Source: CAD feature listing. Evaluate the final solid. Frame: model axes, mm. A direction names the side the tool comes from. Give positions to 0.01 mm unless a question says otherwise; leave off trailing zeros. Return JSON: item names as keys, results as strings. Group by question number.
(1) Access query for faces 1 (the face through (21.5, 2, 22)), 2 (the face through (60, 2, -31)), 3 (the face through (-8, 2, -27.5)), 4 (the face through (-105, 2, -27.5)). Directions: +Z, -Z, +X, -X, +Y, -Y. A direction counts if a zero-diameter tool reaches every point of the face in a straight line with its end or side. Return the directions, or none.
(2) Draft query along Z for faces 5 (the face through (105, 2, 27.5)), 6 (the face through (60, 2, 32)), 7 (the face through (3.859, 2.348, 26.297)). Return one class per face: released by +Z, released by -Z, zero draft, split by the parting line, or undercut.
(3) Cut plane A-A on y = 1.25. Give the number of separate pieces and of enclosed holes in the cut face, then the cut area to 3 significant figures.
(4) Ray query, line 1 (Z direction, x = 56, y = 1.6); line 2 (Z direction, x = -16, y = 4.1); line 3 (X direction, y = 1.85, z = 32.5). Return the intervals inside material, ascending. Write a range as from..to.
(5) Pin query (flat end, axial travel): pin 1 (5 mm diameter, centred on x = 85, z = -5.5, fed in from -Y); pin 2 (1.4 mm diameter, centred on y = 3, z = 35, fed in from -X); pin 3 (2.5 mm diameter, centred on x = -104, y = 3.5, fed in from +Z). Return the tip coordinate at first contact, or that it passes through.
```python
from build123d import *

# Parameters (mm, degrees)
SKETCH1_R           = 1.45
BOSS_EXTRUDE1_DEPTH = 4.7625
SKETCH2_R           = 1.45
SKETCH2_R_2         = 1.6
SKETCH2_R_3         = 2.25
SKETCH2_R_4         = 1.5625
SKETCH2_W           = 25
SKETCH2_H           = 22.5
CUT_EXTRUDE1_DEPTH  = 5.7625
SKETCH3_R           = 0.5
CUT_EXTRUDE2_DEPTH  = 5.7625
FILLET1_R           = 4


with BuildPart() as part:
    # Sketch1 → Boss-Extrude1 (new body)
    with BuildSketch(Plane(origin=(0, 0, 0), x_dir=(1, 0, 0), z_dir=(0, 1, 0))):
        Polygon((100, 37.5), (100, 27.5), (110, 27.5), (110, -27.5), (100, -27.5), (100, -37.5), (-100, -37.5), (-100, -27.5), (-110, -27.5), (-110, 27.5), (-100, 27.5), (-100, 37.5), align=None)
        with Locations((-95, 32.5)):
            Circle(SKETCH1_R, mode=Mode.SUBTRACT)
        with Locations((-105, 22.5)):
            Circle(SKETCH1_R, mode=Mode.SUBTRACT)
        with Locations((105, 22.5)):
            Circle(SKETCH1_R, mode=Mode.SUBTRACT)
        with Locations((95, 32.5)):
            Circle(SKETCH1_R, mode=Mode.SUBTRACT)
        with Locations((-105, -22.5)):
            Circle(SKETCH1_R, mode=Mode.SUBTRACT)
        with Locations((-95, -32.5)):
            Circle(SKETCH1_R, mode=Mode.SUBTRACT)
        with Locations((95, -32.5)):
            Circle(SKETCH1_R, mode=Mode.SUBTRACT)
        with Locations((105, -22.5)):
            Circle(SKETCH1_R, mode=Mode.SUBTRACT)
    extrude(amount=BOSS_EXTRUDE1_DEPTH)

    # Sketch2 → Cut-Extrude1 (cut, through all)
    with BuildSketch(Plane(origin=(0, 4.7625, 0), x_dir=(1, 0, 0), z_dir=(0, 1, 0))):
        with Locations((-25, -22.5)):
            Circle(SKETCH2_R)
        with Locations((-25, 22.5)):
            Circle(SKETCH2_R)
        with Locations((-91.76, -24.96)):
            Circle(SKETCH2_R_2)
        with Locations((-93.03, 23.3)):
            Circle(SKETCH2_R_2)
        with Locations((-40.96, -9.72)):
            Circle(SKETCH2_R_2)
        with Locations((-40.96, 18.22)):
            Circle(SKETCH2_R_2)
        with Locations((45, 5.5)):
            Circle(SKETCH2_R_3)
        with Locations((65, 5.5)):
            Circle(SKETCH2_R_3)
        with Locations((85, 5.5)):
            Circle(SKETCH2_R_3)
        with Locations((56, -21.5)):
            Circle(SKETCH2_R_4)
        with Locations((94, -21.5)):
            Circle(SKETCH2_R_4)
        with Locations((94, 21.5)):
            Circle(SKETCH2_R_4)
        with Locations((56, 21.5)):
            Circle(SKETCH2_R_4)
        Polygon((16.075, 3.65), (23.925, 3.65), (23.925, -7.65), (21.5, -7.65), (21.5, -37.5), (18.5, -37.5), (18.5, -7.65), (16.075, -7.65), align=None)
        with BuildLine():
            Line((70, 37.5), (70, 25.5))
            ThreePointArc((70, 25.5), (65, 20.5), (60, 25.5))
            Line((60, 25.5), (60, 37.5))
            ThreePointArc((60, 37.5), (65, 42.5), (70, 37.5))
        make_face()
        with BuildLine():
            Line((60, -37.5), (60, -25.5))
            ThreePointArc((60, -25.5), (65, -20.5), (70, -25.5))
            Line((70, -25.5), (70, -37.5))
            ThreePointArc((70, -37.5), (65, -42.5), (60, -37.5))
        make_face()
        with Locations((-7.5, -16.25)):
            Rectangle(SKETCH2_W, SKETCH2_H)
        with Locations((-7.5, 16.25)):
            Rectangle(SKETCH2_W, SKETCH2_H)
        with BuildLine():
            Line((-70, -37.5), (-70, -17.5))
            ThreePointArc((-70, -17.5), (-60, -7.5), (-50, -17.5))
            Line((-50, -17.5), (-50, -37.5))
            ThreePointArc((-50, -37.5), (-60, -47.5), (-70, -37.5))
        make_face()
    extrude(amount=-CUT_EXTRUDE1_DEPTH, mode=Mode.SUBTRACT)

    # Sketch3 → Cut-Extrude2 (cut, through all)
    with BuildSketch(Plane(origin=(0, 4.7625, 0), x_dir=(1, 0, 0), z_dir=(0, 1, 0))):
        with Locations((-100.25, 27.75)):
            Circle(SKETCH3_R)
        with Locations((-100.25, -27.75)):
            Circle(SKETCH3_R)
        with Locations((100.25, -27.75)):
            Circle(SKETCH3_R)
        with Locations((100.25, 27.75)):
            Circle(SKETCH3_R)
    extrude(amount=-CUT_EXTRUDE2_DEPTH, mode=Mode.SUBTRACT)

    # Fillet1
    fillet1_edges = [part.edges().sort_by_distance(p)[0] for p in [
        (-20, 2.38125, 27.5),
        (-20, 2.38125, 5),
        (5, 2.38125, 5),
        (5, 2.38125, 27.5),
        (-20, 2.38125, -5),
        (-20, 2.38125, -27.5),
        (5, 2.38125, -27.5),
        (5, 2.38125, -5),
    ]]
    fillet(fillet1_edges, radius=FILLET1_R)


solid = part.part
```
Answers:
{
 "1": {"face 1": "+Z, +Y, -Y", "face 2": "-Z, +Y, -Y", "face 3": "+Y, -Y", "face 4": "-Z, -X, +Y, -Y"},
 "2": {"face 5": "released by +Z", "face 6": "zero draft", "face 7": "undercut"},
 "3": {"separate pieces": "1", "enclosed holes": "23", "area": "13,800 mm²"},
 "4": {"line 1": "-37.5..-23.06, -19.94..19.94, 23.06..37.5", "line 2": "-37.5..-27.5, -5..5, 27.5..37.5", "line 3": "-100..-96.45, -93.55..-70, -50..18.5, 21.5..60, 70..93.55, 96.45..100"},
 "5": {"pin 1": "y = 0", "pin 2": "x = -100", "pin 3": "z = 27.5"}
}
